Part model, mm, in its own coordinate system. Face numbers are marked on the shaded views. Round coordinates to 2 decimals unless told otherwise and drop trailing zeros. Order: outer loops, then holes, each group sorted by start corner. A loop starts at its lowest first (then second) coordinate and runs counter-clockwise, first axis right, second up. Notation, with made-up numbers: M 4.25,65 L 55.25,65 A18 cw 55.25,71 Z; hole C 9.25,74 d11. An arc over 180 degrees is marked long. One line per question, with ' | ' between items.
from build123d import *

# Parameters (mm, degrees)
F0_R     = 19.4183
F0_R_2   = 17.8181
F1_DEPTH = 127
F5_DEPTH = 50.8


with BuildPart() as f1:
    # F0 (on Top) → F1 (new body)
    with BuildSketch(Plane.XY):
        Circle(F0_R)
        Circle(F0_R_2, mode=Mode.SUBTRACT)
    extrude(amount=F1_DEPTH)

    # F4 (on face) → F5 (cut, symmetric)
    with BuildSketch(Plane(origin=(0, 19.4183, 0), x_dir=(-1, 0, 0), z_dir=(0, 1, 0))):
        with BuildLine():
            ThreePointArc((0, 116.078), (-1.257236, 113.042764), (1.778, 114.3))
            ThreePointArc((1.778, 114.3), (1.257236, 115.557236), (0, 116.078))
        make_face()
    extrude(amount=F5_DEPTH, both=True, mode=Mode.SUBTRACT)


solid = f1.part
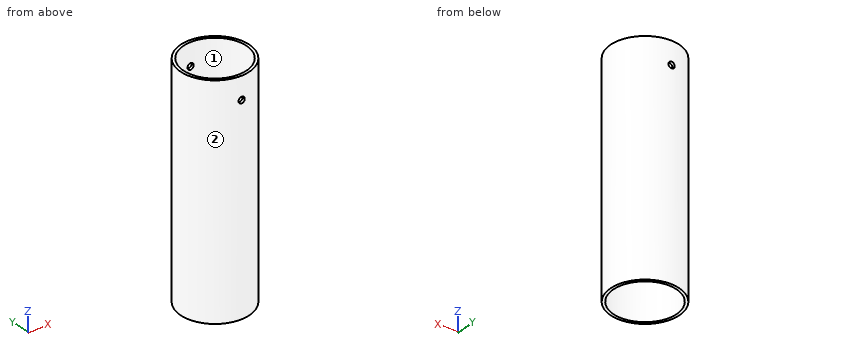
1) Saw through at C-C (z = 38). List the corners of the cut face in (x, y).
The answers:
outline: C 0,0 d38.84; hole C 0,0 d35.64
2) Drop flat-ended pins along their axis: pin 1 (1 mm diameter, centred on x = 10, z = 50.5, fed in from +Y); pin 2 (3 mm diameter, centred on x = 7, z = 50, fed in from -Y); pin 3 (4 mm diameter, centred on x = -2.5, z = 52.5, fed in from +Y); pin 4 (2 mm diameter, centred on x = 0, z = 114.3, fed in from +Y). Give the stop position or say it passes through.
The answers:
pin 1: stops at y = 16.94 | pin 2: stops at y = -18.62 | pin 3: stops at y = 19.41 | pin 4: passes through
3) Two-plate mould, pull along X, no slides. Class the marked faces 1 and 2: released by +X, released by -X, zero draft, split by the parting line, or undercut.
The answers:
face 1: undercut | face 2: split by the parting line
4) Saw through at A-A (y = 0). List the corners of the cut face in (x, z).
The answers:
outline: M -19.42,0 L -17.82,0 L -17.82,127 L -19.42,127 Z; M 17.82,0 L 19.42,0 L 19.42,127 L 17.82,127 Z
5) Saw through at B-B (x = -10). List the corners of the cut face in (y, z), plus the area to 3 significant figures.
The answers:
outline: M -16.65,0 L -14.75,0 L -14.75,127 L -16.65,127 Z; M 14.75,0 L 16.65,0 L 16.65,127 L 14.75,127 Z | area: 482 mm²
6) Probe line 1 (X direction, y = -10, z = 72.5); line 2 (X direction, y = 12.5, z = 52.5); line 3 (Y direction, x = 13, z = 85). List the from-to ranges inside material, lowest first. Write a range as [from, to].
The answers:
line 1: x = [-16.65, -14.75], [14.75, 16.65] | line 2: x = [-14.86, -12.7], [12.7, 14.86] | line 3: y = [-14.42, -12.19], [12.19, 14.42]
